Could you check a few things on this model? Use its own coordinates, in mm. Face numbers are marked on the shaded views. A direction names the side the tool comes from. Round coordinates to 2 decimals unless told otherwise and drop trailing zeros. Loops run counter-clockwise (first coordinate to the right, second up) from the corner with the lowest first, then second, coordinate; pieces in that order, holes last. Notation, with made-up numbers: M 74,-20.75 L 102,-20.75 A24 ccw 102,15.25 Z; hole C 59.5,-21.5 d1. An arc over 180 degrees is marked long. Return JSON: item names as keys, results as strings. Group by question number.
```python
from build123d import *
from OCP.BRepFilletAPI import BRepFilletAPI_MakeChamfer

# Parameters (mm, degrees)
SKETCH_1_W          = 370
SKETCH_1_H          = 70
EXTRUDE_1_DEPTH     = 10
SKETCH_2_W          = 350
SKETCH_2_H          = 50
EXTRUDE_2_DEPTH     = 10
SKETCH_3_W          = 350
SKETCH_3_H          = 50
EXTRUDE_3_DEPTH     = 200
CHAMFER_1_SIZE      = 112
CHAMFER_1_SIZE2     = 152
SHELL_START         = -20
SHELL_1_DEPTH       = 40
SKETCH_4_R          = 12.5
CUT_EXTRUDE_1_DEPTH = 30


# Read off the part's stored shape, not the designer's step: 抽壳1
with BuildPart() as part:
    # 草图1 → 凸台-拉伸1 (new body)
    with BuildSketch(Plane(origin=(0, 0, 0), x_dir=(1, 0, 0), z_dir=(0, 1, 0))):
        Rectangle(SKETCH_1_W, SKETCH_1_H)
    extrude(amount=EXTRUDE_1_DEPTH)

    # 草图2 → 凸台-拉伸2 (add)
    with BuildSketch(Plane(origin=(0, 10, 0), x_dir=(1, 0, 0), z_dir=(0, 1, 0))):
        Rectangle(SKETCH_2_W, SKETCH_2_H)
    extrude(amount=EXTRUDE_2_DEPTH)

    # 草图3 → 凸台-拉伸3 (add)
    with BuildSketch(Plane.XZ):
        Rectangle(SKETCH_3_W, SKETCH_3_H)
    extrude(amount=EXTRUDE_3_DEPTH)

    # 倒角1: one chamfer whose edges measure the first distance from different faces: ONE call of the kernel's chamfer builder (chamfer() names one face for all edges)
    chamfer_1_edges_1 = [part.edges().sort_by_distance(p)[0] for p in [
        (-175, -200, 0),
    ]]
    chamfer_1_side_1 = [part.faces().sort_by_distance(p)[0] for p in [
        (-175, -100, 0),
    ]]
    chamfer_1_edges_2 = [part.edges().sort_by_distance(p)[0] for p in [
        (175, -200, 0),
    ]]
    chamfer_1_side_2 = [part.faces().sort_by_distance(p)[0] for p in [
        (175, -100, 0),
    ]]
    chamfer_1 = BRepFilletAPI_MakeChamfer(part.part.solid().wrapped)
    for e in chamfer_1_edges_1:
        chamfer_1.Add(CHAMFER_1_SIZE, CHAMFER_1_SIZE2, e.wrapped, chamfer_1_side_1[0].wrapped)  # the first distance lies on this face
    for e in chamfer_1_edges_2:
        chamfer_1.Add(CHAMFER_1_SIZE, CHAMFER_1_SIZE2, e.wrapped, chamfer_1_side_2[0].wrapped)  # the first distance lies on this face
    add(Compound.cast(chamfer_1.Shape()), mode=Mode.REPLACE)

    # 抽壳1 outline → 抽壳1 (cut)
    with BuildSketch(Plane.XY.offset(SHELL_START)):
        Polygon((170, -85.473461199), (170, 20), (-170, 20), (-170, -85.473461199), (-21.356840199, -195), (21.356840199, -195), align=None)
    extrude(amount=SHELL_1_DEPTH, mode=Mode.SUBTRACT)

    # 草图4 → 切除-拉伸1 (cut)
    with BuildSketch(Plane.XZ.offset(200)):
        with Locations(Location((0, 0, 0), (0, 0, 270))):
            Circle(SKETCH_4_R)
    extrude(amount=-CUT_EXTRUDE_1_DEPTH, mode=Mode.SUBTRACT)


solid = part.part
```
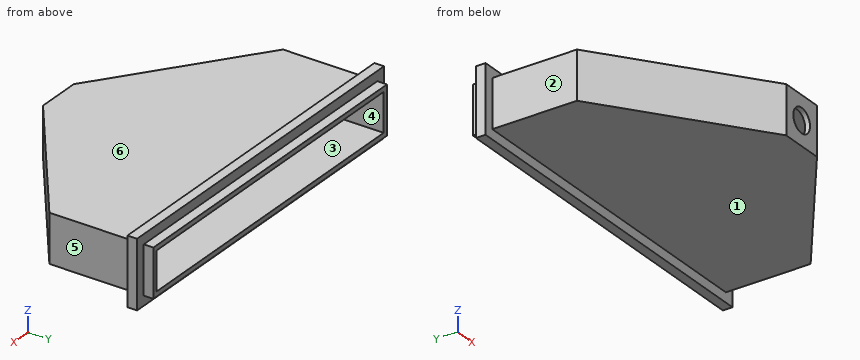
1. If we section it at D-D, the plane y = 5: Please give me the cut outline in (x, z).
2. If we section it at C-C, the plane x = 0: Please give me the cut outline in (y, z), then the cut area to 4 significant figures.
3. I'm going to push flat-ended pins straight in: pin 1 Ø6 at (y, z) = (-111.5, 24) entering from +X; pin 2 Ø2 at (x, z) = (-95.5, -8.5) entering from +Y; pin 3 Ø3 at (y, z) = (-134, -3.5) entering from -X. Where does each tip first touch, or does it pass through?
4. If we section it at A-A, the plane y = -71: Please give me the cut outline in (x, z), then the cut area to 3 significant figures.
5. If we section it at B-B, the plane z = 0: Please give me the cut outline in (x, y).
6. On a 3-axis mill with a long thin cutter (end or side, diameter ignored), from which of +Z, -Z, +X, -X, +Y, -Y can I reach the whole of each face in a straight line? I mean the marked faces 1 and 2. Say none if no direction works.
7. We'd pull the mould along Z, two halves only. Please class the marked faces 3, 4, 5 and 6: +Z half, -Z half, draft (parallel to the pull), parting line (faces both ways), or undercut.
8. I need wall thicknesses on probe 1 along X at (y, z) = (-71, -13.5); probe 2 along Z at (x, y) = (45, -83.5); probe 3 along Y at (x, z) = (126, 30.5). Which ranges of each line are inside material? Lowest first, please.
Geometry results:
{
 "1": {"outline": "M -185,-35 L 185,-35 L 185,35 L -185,35 Z; hole M -170,-20 L 170,-20 L 170,20 L -170,20 Z"},
 "2": {"outline": "M -200,-25 L 0,-25 L 0,-35 L 10,-35 L 10,-25 L 20,-25 L 20,-20 L -195,-20 L -195,-12.5 L -200,-12.5 Z; M -200,12.5 L -195,12.5 L -195,20 L 20,20 L 20,25 L 10,25 L 10,35 L 0,35 L 0,25 L -200,25 Z", "area": "2,475 mm^2"},
 "3": {"pin 1": "x = 147.18", "pin 2": "y = -139.63", "pin 3": "x = -114.61"},
 "4": {"outline": "M -175,-25 L 175,-25 L 175,25 L -175,25 Z; hole M -170,-20 L 170,-20 L 170,20 L -170,20 Z", "area": "3,900 mm^2"},
 "5": {"outline": "M -185,0 L -175,0 L -175,-88 L -23,-200 L -12.5,-200 L -12.5,-195 L -21.36,-195 L -170,-85.47 L -170,20 L -175,20 L -175,10 L -185,10 Z; M 12.5,-200 L 23,-200 L 175,-88 L 175,0 L 185,0 L 185,10 L 175,10 L 175,20 L 170,20 L 170,-85.47 L 21.36,-195 L 12.5,-195 Z"},
 "6": {"face 1": "-Z, +X, -X, -Y", "face 2": "+Z, -Z, -X, -Y"},
 "7": {"face 3": "undercut", "face 4": "undercut", "face 5": "draft", "face 6": "+Z half"},
 "8": {"probe 1": "-175 to -170, 170 to 175", "probe 2": "-25 to -20, 20 to 25", "probe 3": "0 to 10"}
}
